from build123d import *

# Parameters (mm, degrees)
SKETCH1_W           = 45
SKETCH1_H           = 28
BOSS_EXTRUDE1_DEPTH = 3
BOSS_EXTRUDE2_DEPTH = 22
SKETCH4_W           = 45
SKETCH4_H           = 28
SKETCH4_W_2         = 3
SKETCH4_H_2         = 24
BOSS_EXTRUDE4_DEPTH = 2
SKETCH5_W           = 9
SKETCH5_H           = 4
CUT_EXTRUDE1_DEPTH  = 2
SKETCH6_W           = 3
SKETCH6_H           = 24
CUT_EXTRUDE2_DEPTH  = 3
SKETCH7_W           = 45
SKETCH7_H           = 28
SKETCH7_W_2         = 3
SKETCH7_H_2         = 24
BOSS_EXTRUDE5_DEPTH = 1


with BuildPart() as part:
    # Sketch1 → Boss-Extrude1 (new body)
    with BuildSketch(Plane(origin=(0, 0, 0), x_dir=(1, 0, 0), z_dir=(0, 1, 0))):
        with Locations((22.5, 14)):
            Rectangle(SKETCH1_W, SKETCH1_H)
    extrude(amount=BOSS_EXTRUDE1_DEPTH)

    # Sketch2 → Boss-Extrude2 (add)
    with BuildSketch(Plane(origin=(0, 3, 0), x_dir=(1, 0, 0), z_dir=(0, 1, 0))):
        Polygon((40, 26), (40, 28), (0, 28), (0, 0), (40, 0), (40, 2), (2, 2), (2, 26), align=None)
    extrude(amount=BOSS_EXTRUDE2_DEPTH)

    # Sketch4 → Boss-Extrude4 (add)
    with BuildSketch(Plane(origin=(0, 25, 0), x_dir=(1, 0, 0), z_dir=(0, 1, 0))):
        with Locations((22.5, 14)):
            Rectangle(SKETCH4_W, SKETCH4_H)
        with Locations((41.5, 14)):
            Rectangle(SKETCH4_W_2, SKETCH4_H_2, mode=Mode.SUBTRACT)
    extrude(amount=-BOSS_EXTRUDE4_DEPTH)

    # Sketch5 → Cut-Extrude1 (cut)
    with BuildSketch(Plane.ZY):
        with BuildLine():
            Line((-18.72, 5.25), (-18.72, 6.16))
            ThreePointArc((-18.72, 6.16), (-18.353883476, 7.043883476), (-17.47, 7.41))
            Line((-17.47, 7.41), (-10.53, 7.41))
            ThreePointArc((-10.53, 7.41), (-9.646116524, 7.043883476), (-9.28, 6.16))
            Line((-9.28, 6.16), (-9.28, 5.25))
            ThreePointArc((-9.28, 5.25), (-9.646116524, 4.366116524), (-10.53, 4))
            Line((-10.53, 4), (-17.47, 4))
            ThreePointArc((-17.47, 4), (-18.353883476, 4.366116524), (-18.72, 5.25))
        make_face()
        with Locations((-14, 10.5)):
            Rectangle(SKETCH5_W, SKETCH5_H)
    extrude(amount=-CUT_EXTRUDE1_DEPTH, mode=Mode.SUBTRACT)

    # Sketch6 → Cut-Extrude2 (cut)
    with BuildSketch(Plane(origin=(0, 3, 0), x_dir=(1, 0, 0), z_dir=(0, 1, 0))):
        with Locations((41.5, 14)):
            Rectangle(SKETCH6_W, SKETCH6_H)
    extrude(amount=-CUT_EXTRUDE2_DEPTH, mode=Mode.SUBTRACT)

    # Sketch7 → Boss-Extrude5 (add)
    with BuildSketch(Plane(origin=(0, 25, 0), x_dir=(1, 0, 0), z_dir=(0, 1, 0))):
        with Locations((22.5, 14)):
            Rectangle(SKETCH7_W, SKETCH7_H)
        with Locations((41.5, 14)):
            Rectangle(SKETCH7_W_2, SKETCH7_H_2, mode=Mode.SUBTRACT)
    extrude(amount=BOSS_EXTRUDE5_DEPTH)


solid = part.part
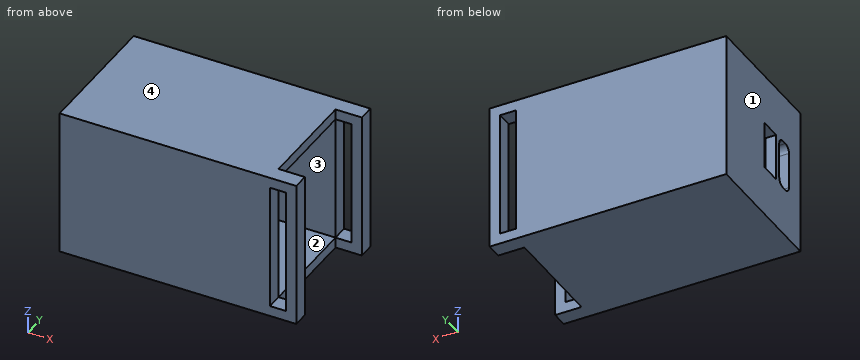
Source: CAD feature listing. Evaluate the final solid. Frame: model axes, mm. Face numbers are marked on the shaded views. Give positions to 0.01 mm unless a question says otherwise; leave off trailing zeros. Write each loop counter-clockwise with the first axis right and the second up, starting at its lowest first coordinate (ties: lowest second). Pieces come first, ordered by that corner, then holes. Notation, with made-up numbers: M 25.25,65.5 L 53.25,65.5 A22 ccw 53.25,82.5 Z; hole C -35.75,-31 d5. An arc over 180 degrees is marked long. Return JSON: item names as keys, results as strings. Group by question number.
1) Pull-direction query (Z, two-part tool) for the marked faces 1, 2, 3 and 4; classes: pulls with the +Z half, pulls with the -Z half, needs draft (parallel to the pull), parting line crosses it, or undercut.
2) Cut plane B-B, the plane x = 23. Output: boundary loops of the cut face in (y, z).
3) Cut plane C-C, the plane y = 24. Output: boundary loops of the cut face in (x, z), plus the area to 3 significant figures.
4) Material intervals for line 1 along Z through (x, y) = (15.5, 20.25); line 2 along Y through (x, z) = (21.5, -22.25); line 3 along X through (y, z) = (2.5, -25), sorted ascending. Write a range as [from, to].
5) Cut plane A-A, the plane y = 10.5. Output: boundary loops of the cut face in (x, z).
6) Pin query (flat end, axial travel): P1, Ø3.5, axis at x = 41, y = 24.5, coming from the +Z side; P2, Ø6, axis at y = 11, z = -15.5, coming from the +X side; P3, Ø1, axis at y = 8.5, z = -26.5, coming from the +X side. Return the tip coordinate at first contact, or that it passes through.
7) Cut plane D-D, the plane z = -13.25. Output: boundary loops of the cut face in (x, y).
Recorded:
{
 "1": {"face 1": "needs draft", "face 2": "undercut", "face 3": "undercut", "face 4": "pulls with the +Z half"},
 "2": {"outline": "M 0,-28 L 26,-28 L 26,0 L 0,0 Z; hole M 3,-26 L 23,-26 L 23,-2 L 3,-2 Z"},
 "3": {"outline": "M 0,-28 L 45,-28 L 45,0 L 0,0 Z; hole M 40,-26 L 43,-26 L 43,-2 L 40,-2 Z", "area": "1,190 mm²"},
 "4": {"line 1": "z = [-28, -26], [-2, 0]", "line 2": "y = [0, 3], [23, 26]", "line 3": "x = [0, 40], [43, 45]"},
 "5": {"outline": "M 0,-28 L 40,-28 L 40,-26 L 2,-26 L 2,-18.5 L 0,-18.5 Z; M 0,-9.5 L 2,-9.5 L 2,-2 L 40,-2 L 40,0 L 0,0 Z"},
 "6": {"P1": "stops at z = 0", "P2": "stops at x = 2", "P3": "stops at x = 40"},
 "7": {"outline": "M 0,0 L 40,0 L 40,3 L 2,3 L 2,4 L 0,4 Z; M 0,7.41 L 2,7.41 L 2,8.5 L 0,8.5 Z; M 0,12.5 L 2,12.5 L 2,23 L 40,23 L 40,26 L 0,26 Z; M 43,0 L 45,0 L 45,3 L 43,3 Z; M 43,23 L 45,23 L 45,26 L 43,26 Z"}
}
